```python
from build123d import *

# Parameters (mm, degrees)
F0_W     = 210
F0_H     = 375
F0_R     = 12
F0_R_2   = 35
F1_DEPTH = 10


with BuildPart() as f1:
    # F0 (on Front) → F1 (new body, symmetric)
    with BuildSketch(Plane.XZ):
        Rectangle(F0_W, F0_H)
        with Locations((-48, -132.5)):
            Circle(F0_R, mode=Mode.SUBTRACT)
        with Locations((-48, -67.5)):
            Circle(F0_R, mode=Mode.SUBTRACT)
        with Locations((48, -132.5)):
            Circle(F0_R, mode=Mode.SUBTRACT)
        with Locations((48, -67.5)):
            Circle(F0_R, mode=Mode.SUBTRACT)
        with Locations((0, 107.5)):
            Circle(F0_R_2, mode=Mode.SUBTRACT)
    extrude(amount=F1_DEPTH, both=True)


solid = f1.part
```
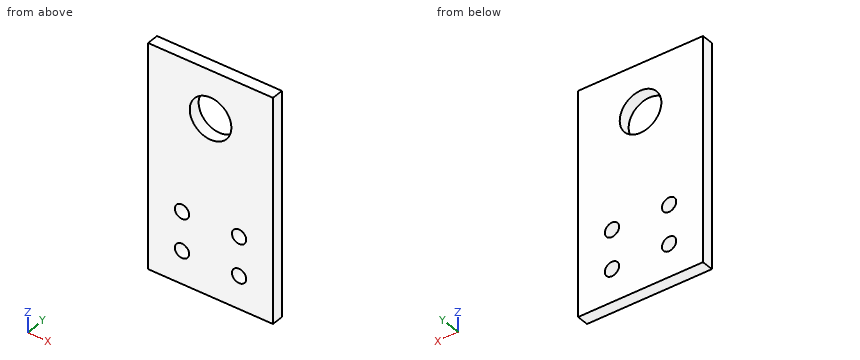
Check sheet for the modelled part. Datum: model origin and axes. Units: mm. Round coordinates to 2 decimals unless told otherwise and drop trailing zeros. Order: outer loops, then holes, each group sorted by start corner. A loop starts at its lowest first (then second) coordinate and runs counter-clockwise, first axis right, second up. Notation, with made-up numbers: (25.25, -0.5) - (65.25, -0.5) arc R27 cw to (65.25, 15.5) - close; hole circle Ø6 at (59, 21.5). An arc over 180 degrees is marked (long way). Answer as CSV lines item,"result". Start each with the question number.
1) Section check A-A (z = 107.5). Record the cut outline in (x, y), then the cut area to 3 significant figures.
2) Section check C-C (y = 0). Record the cut outline in (x, z), then the cut area to 3 significant figures.
3) Section check D-D (z = -67.5). Record the cut outline in (x, y), then the cut area to 3 significant figures.
4) Scan lines: probe 1 along Z at (x, y) = (48, -5.25); probe 2 along Z at (x, y) = (0, -3.5); probe 3 along Z at (x, y) = (18, 3.5). Record each from-to range of solid material in increasing order.
5) Section check B-B (x = 0). Record the cut outline in (y, z), then the cut area to 3 significant figures.
6) Depth check by flat-ended pin: pin 1 (21.5 mm diameter, centred on x = 48, z = -132.5, fed in from +Y). Enter the tip coordinate at first touch or a pass-through.
Determined:
1,outline,"(-105, -10) - (-35, -10) - (-35, 10) - (-105, 10) - close; (35, -10) - (105, -10) - (105, 10) - (35, 10) - close"
1,area,"2,800 mm^2"
2,outline,"(-105, -187.5) - (105, -187.5) - (105, 187.5) - (-105, 187.5) - close; hole circle Ø24 at (-48, -132.5); hole circle Ø24 at (-48, -67.5); hole circle Ø70 at (0, 107.5); hole circle Ø24 at (48, -132.5); hole circle Ø24 at (48, -67.5)"
2,area,"73,100 mm^2"
3,outline,"(-105, -10) - (-60, -10) - (-60, 10) - (-105, 10) - close; (-36, -10) - (36, -10) - (36, 10) - (-36, 10) - close; (60, -10) - (105, -10) - (105, 10) - (60, 10) - close"
3,area,"3,240 mm^2"
4,probe 1,"-187.5 to -144.5, -120.5 to -79.5, -55.5 to 187.5"
4,probe 2,"-187.5 to 72.5, 142.5 to 187.5"
4,probe 3,"-187.5 to 77.48, 137.52 to 187.5"
5,outline,"(-10, -187.5) - (10, -187.5) - (10, 72.5) - (-10, 72.5) - close; (-10, 142.5) - (10, 142.5) - (10, 187.5) - (-10, 187.5) - close"
5,area,"6,100 mm^2"
6,pin 1,"through"
